Autodesk Inventor part; units mm, degrees
ref_plane "YZ Plane" through (0, 0, 0) normal (1, 0, 0) x (0, 1, 0)
ref_plane "XZ Plane" through (0, 0, 0) normal (0, 1, 0) x (-1, 0, 0)
ref_plane "XY Plane" through (0, 0, 0) normal (0, 0, 1) x (1, 0, 0)
sketch "Sketch1" plane through (0, 0, 0) normal (0, 0, 1) x (1, 0, 0)
  line L0 (0, 0) -> (-100, 0)
  line L1 (-100, 20) -> (0, 20)
  line L2 (0, 20) -> (0, 0)
  line L3 (-100, 20) -> (-220, 10)
  line L4 (-220, 10) -> (-100, 0)
  line L5 (-25, 25) -> (-10, 25)
  line L6 (-10, 25) -> (-10, 20)
  line L7 (-10, 20) -> (-25, 20)
  line L8 (-25, 20) -> (-25, 25)
  line L9 (-25, 0) -> (-10, 0)
  line L10 (-10, 0) -> (-10, -5)
  line L11 (-10, -5) -> (-25, -5)
  line L12 (-25, -5) -> (-25, 0)
  dimension "d0" = 100
  dimension "d1" = 20
  dimension "d2" = 220
  dimension "d3" = 10
  dimension "d4" = 15
  dimension "d5" = 5
  dimension "d6" = 10
extrude "Cuerpo" add sketch "Sketch1" along normal blind 3
sketch "Sketch2" plane through (0, 0, 0) normal (0, 0, -1) x (-1, 0, 0)
  line L0 (0, 0) -> (0, 20)
  line L1 (100, 20) -> (220, 10)
  line L2 (220, 10) -> (100, 0)
  line L3 (190, 7.5) -> (0, 7.5)
  line L4 (190, 12.5) -> (0, 12.5)
  dimension "d9" = 5
extrude "Rail" add sketch "Sketch2" along normal blind 1
draft "FaceDraft1" angle -20 pull direction (0, 0, 1) faces at (-25, -1.6667, 1) fixed edges at (-25, -2.5, 0)
draft "FaceDraft2" angle -20 pull direction (0, 0, 1) faces at (-10, -3.3333, 1) fixed edges at (-10, -2.5, 0)
draft "FaceDraft3" angle -20 pull direction (0, 0, 1) faces at (-10, 21.6667, 1) fixed edges at (-10, 22.5, 0)
draft "FaceDraft4" angle -20 pull direction (0, 0, 1) faces at (-25, 23.3333, 1) fixed edges at (-25, 22.5, 0)
equation "\"d0\" = hoja_cuerpo_largo"
equation "\"d1\" = hoja_ancho"
equation "\"d2\" = hoja_largo"
equation "\"d3\" = hoja_diente_separacion"
equation "\"d4\" = hoja_diente_largo"
equation "\"d5\" = hoja_diente_ancho"
equation "\"d6\" = d3"
equation "\"d7\" = hoja_grosor"
equation "\"d9\" = hoja_rail_ancho"
equation "\"d10\" = hoja_rail_alto"
equation "\"d12\" = tirador_diente_agarre"
equation "\"d13\" = tirador_diente_agarre"
equation "\"d14\" = tirador_diente_agarre"
equation "\"d15\" = tirador_diente_agarre"
properties part number "Hoja"
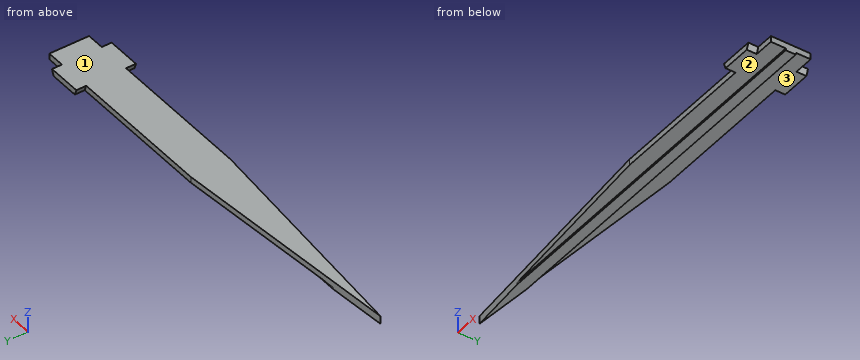
CAD build for the part. Positions are in the model's coordinates, mm. Face numbers are marked on the shaded views. A direction names the side the tool comes from. Give positions to 0.01 mm unless a question says otherwise; leave off trailing zeros. Order: outer loops, then holes, each group sorted by start corner. A loop starts at its lowest first (then second) coordinate and runs counter-clockwise, first axis right, second up.
(1) Drill centre lines: L1, parallel to Z at x = -51, y = 18.5; L2, parallel to Y at x = -98, z = 0.5; L3, parallel to Y at x = -99, z = -0.2. Where is each one in solid material? Low to high.
(2) Saw through at D-D, the plane x = -142. Give the cut face in (y, z), then the cut area to 3 significant figures.
(3) Saw through at C-C, the plane y = 4. Give the cut face in (x, z).
(4) Saw through at A-A, the plane x = -46. Give the cut face in (y, z).
(5) Flat gauge pins, fed straight in: pin 1 (0.9 mm diameter, centred on x = -54.5, z = 1, fed in from +Y); pin 2 (1.5 mm diameter, centred on x = -63, z = 1.5, fed in from -Y); pin 3 (1.1 mm diameter, centred on x = -103.5, z = -0.5, fed in from +Y). Where does each tip first touch, or does it go through?
(6) Saw through at B-B, the plane z = 0.65. Give the cut face in (x, y), then the cut area to 3 significant figures.
(7) Tool access for the marked faces 1, 2 and 3: list every direction of +Z, -Z, +X, -X, +Y, -Y with a clear straight run to the whole face (end or side of a thin tool).
Results found:
1. L1: z = 0 to 3
1. L2: y = 0 to 20
1. L3: y = 7.5 to 12.5
2. outline: (3.5, 0) - (7.5, 0) - (7.5, -1) - (12.5, -1) - (12.5, 0) - (16.5, 0) - (16.5, 3) - (3.5, 3) - close
2. area: 44.0 mm2
3. outline: (-148, 0) - (0, 0) - (0, 3) - (-148, 3) - close
4. outline: (0, 0) - (7.5, 0) - (7.5, -1) - (12.5, -1) - (12.5, 0) - (20, 0) - (20, 3) - (0, 3) - close
5. pin 1: stops at y = 20
5. pin 2: stops at y = 0
5. pin 3: stops at y = 19.73
6. outline: (-220, 10) - (-100, 0) - (-25.24, 0) - (-25.24, -5) - (-9.76, -5) - (-9.76, 0) - (0, 0) - (0, 20) - (-9.76, 20) - (-9.76, 25) - (-25.24, 25) - (-25.24, 20) - (-100, 20) - close
6. area: 3,350 mm2
7. face 1: +Z, +X, -X, +Y, -Y
7. face 2: -Z, +X, -X, -Y
7. face 3: -Z, +X, -X, +Y
